Geometry check sheet. Reference: drawing and pictorial views, mm from the part's lowest x, y, z. Round coordinates to 2 decimals unless told otherwise and drop trailing zeros. Write each loop counter-clockwise with the first axis right and the second up, starting at its lowest first coordinate (ties: lowest second). Pieces come first, ordered by that corner, then holes. Notation, with made-up numbers: (-3.5, -29.5) - (17.5, -29.5) arc R11 ccw to (17.5, -10.5) - close; hole circle Ø9 at (0, 27). An arc over 180 degrees is marked (long way). Use one line per item in the form item = value. Start each with the question number.
1) Section check C-C (x = 7). Record the boundary of the cut face in (y, z) (1 decimal).
2) Draft check along X on the marked faces 1, 2 and 3. Enter one of: +X half, -X half, draft (parallel to the pull), parting line (faces both ways), or undercut.
3) Section check A-A (z = 3.75). Record the boundary of the cut face in (x, y) (1 decimal).
4) Section check D-D (x = 2). Record the boundary of the cut face in (y, z), then the cut area to 3 significant figures.
5) Gauge pin test, flat ends, axial feed: P1, Ø1.5, axis at y = 2.5, z = 11.5, coming from the +X side; P2, Ø1, axis at y = 4.5, z = 11.5, coming from the -X side; P3, Ø1.5, axis at x = 12, y = 4, coming from the -Z side. Record the tip position at first contact, or that the pin passes through.
6) Section check B-B (y = 4.6). Record the boundary of the cut face in (x, z) (1 decimal).
7) Scan lines: probe 1 along X at (y, z) = (3.4, 5.25) (1 decimal); probe 2 along Z at (x, y) = (8, 2) (1 decimal); probe 3 along Z at (x, y) = (8.5, 0.45) (1 decimal). Record each from-to range of solid material in increasing order.
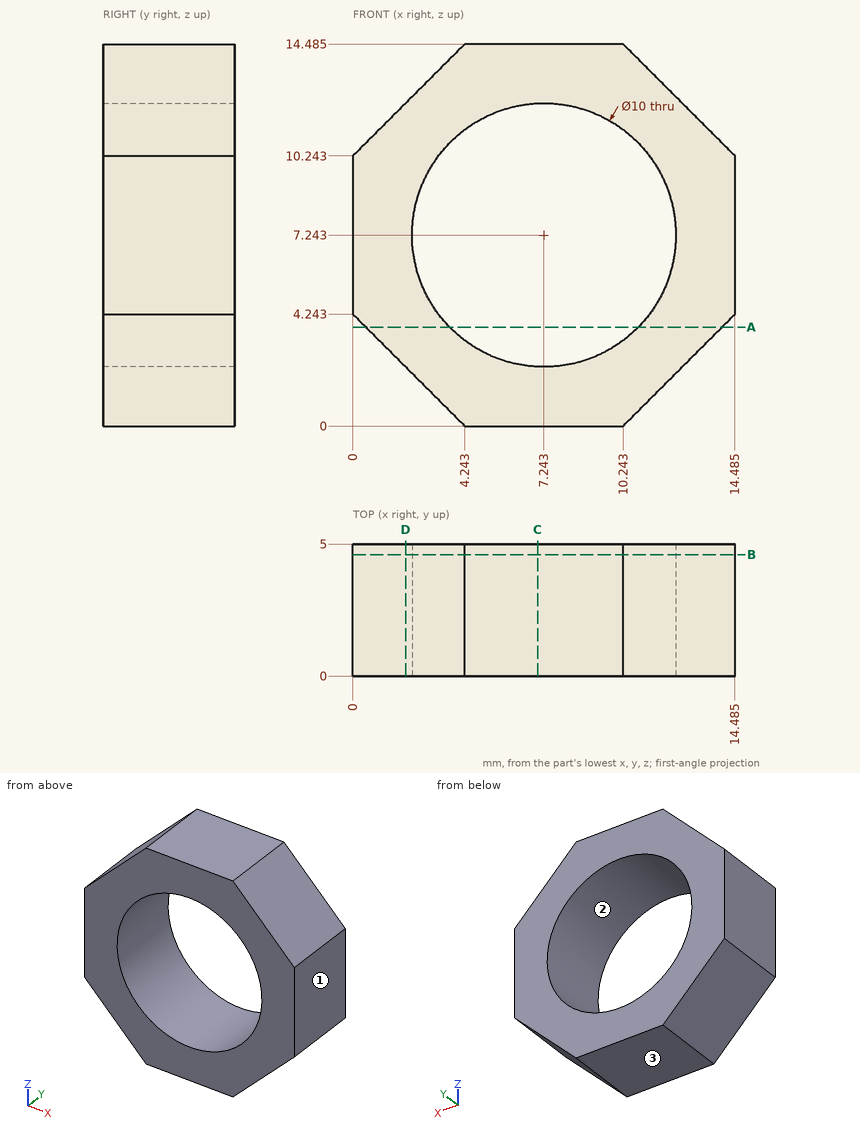
Results are:
q1.outline = (0, 0) - (5, 0) - (5, 2.2) - (0, 2.2) - close; (0, 12.2) - (5, 12.2) - (5, 14.5) - (0, 14.5) - close
q2.face_1 = +X half
q2.face_2 = undercut
q2.face_3 = draft
q3.outline = (0.5, 0) - (3.7, 0) - (3.7, 5) - (0.5, 5) - close; (10.8, 0) - (14, 0) - (14, 5) - (10.8, 5) - close
q4.outline = (0, 2.24) - (5, 2.24) - (5, 12.24) - (0, 12.24) - close
q4.area = 50.0 mm²
q5.P1 = 13.98
q5.P2 = 0.76
q5.P3 = 1.01
q6.outline = (0, 4.2) - (4.2, 0) - (10.2, 0) - (14.5, 4.2) - (14.5, 10.2) - (10.2, 14.5) - (4.2, 14.5) - (0, 10.2) - close; hole circle Ø10 at (7.2, 7.2)
q7.probe_1 = 0 to 2.7, 11.8 to 14.5
q7.probe_2 = 0 to 2.3, 12.2 to 14.5
q7.probe_3 = 0 to 2.4, 12.1 to 14.5
